Could you check a few things on this drawing? It's one solid part, dimensions in mm from its lowest x, y, z. A direction names the side the tool comes from. Give positions to 0.01 mm unless a question says otherwise; leave off trailing zeros. Write each loop counter-clockwise with the first axis right and the second up, starting at its lowest first coordinate (ties: lowest second). Pieces come first, ordered by that corner, then holes. Notation, with made-up numbers: M 64.25,-36.5 L 76.25,-36.5 A22 cw 76.25,-30.5 Z; hole C 62.5,-29.5 d1. An arc over 180 degrees is marked long. Write each question's results on one line, items separated by ' | '.
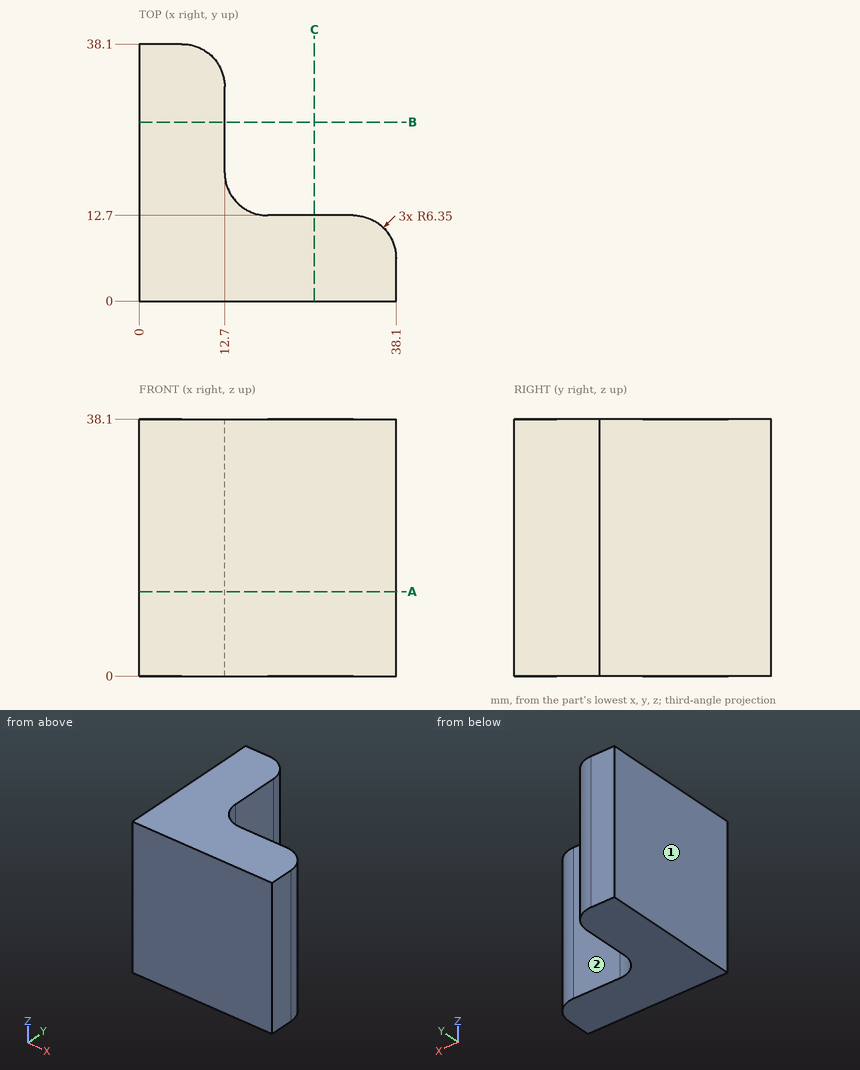
Item 1: I want a section at A-A, the plane z = 12.5. Please give me the cut outline in (x, y).
Geometry says:
outline: M 0,0 L 38.1,0 L 38.1,6.35 A6.35 ccw 31.75,12.7 L 19.05,12.7 A6.35 cw 12.7,19.05 L 12.7,31.75 A6.35 ccw 6.35,38.1 L 0,38.1 Z
Item 2: I'm going to push flat-ended pins straight in: pin 1 (6 mm diameter, centred on y = 26, z = 15, fed in from +X); pin 2 (6.5 mm diameter, centred on x = 28, z = 17.5, fed in from +Y). Where does each tip first touch, or does it pass through?
Geometry says:
pin 1: stops at x = 12.7 | pin 2: stops at y = 12.7
Item 3: For the marked faces 1 and 2, which set-ups out of +Z, -Z, +X, -X, +Y, -Y let a thin tool reach every point of the face, with its end or its side?
Geometry says:
face 1: +Z, -Z, -X, +Y, -Y | face 2: +Z, -Z, +X, +Y
Item 4: If I drill on line 1 (Y direction, x = 6.5, z = 25); line 2 (Y direction, x = 29, z = 17.5), over which ranges is the centre line in solid material (lowest first)? Write a range as from..to.
Geometry says:
line 1: y = 0..38.1 | line 2: y = 0..12.7
Item 5: I want a section at B-B, the plane y = 26.5. Please give me the cut outline in (x, z), and give its area (3 significant figures).
Geometry says:
outline: M 0,0 L 12.7,0 L 12.7,38.1 L 0,38.1 Z | area: 484 mm2
